Autodesk Inventor part; units mm, degrees
ref_plane "YZ Plane" through (0, 0, 0) normal (1, 0, 0) x (0, 1, 0)
ref_plane "XZ Plane" through (0, 0, 0) normal (0, 1, 0) x (-1, 0, 0)
ref_plane "XY Plane" through (0, 0, 0) normal (0, 0, 1) x (1, 0, 0)
sketch "Sketch1" plane through (0, 0, 0) normal (0, 0, 1) x (1, 0, 0)
  line L0 (0, 39.36) -> (0, -6.56)
  line L1 (-29.4, 0) -> (29.4, 0)
  line L2 (-21, 0) -> (21, 0)
  line L3 (21, 0) -> (21, 6)
  line L4 (21, 6) -> (9, 6)
  line L5 (9, 6) -> (9, 32.8)
  line L6 (9, 32.8) -> (0.5, 32.8)
  line L7 (0.5, 32.8) -> (0.5, 23.9686)
  line L8 (-0.5, 23.9686) -> (-0.5, 32.8)
  line L9 (-0.5, 32.8) -> (-9, 32.8)
  line L10 (-9, 32.8) -> (-9, 6)
  line L11 (-9, 6) -> (-21, 6)
  line L12 (-21, 6) -> (-21, 0)
  circle A0 centre (0, 20) radius 4
  point P0 (0, 0)
  dimension "d0" = 42
  dimension "d1" = 6
  dimension "d2" = 20
  dimension "d3" = 32.8
  dimension "d4" = 21
  dimension "d5" = 18
  dimension "d6" = 8
  dimension "d7" = 1
extrude "Extrusion1" add sketch "Sketch1" along normal mid plane 14 contours A0 L7 L6 L5 L4 L3 L1 L0 | L0 L1 L12 L11 L10 L9 L8 A0
sketch "Sketch2" plane through (-21, 6, -7) normal (0, 1, 0) x (1, 0, 0)
  line L0 (0, 0) -> (12, 0)
  line L1 (0, 0) -> (0, -14)
  line L2 (12, -14) -> (0, -14)
  line L3 (12, 0) -> (12, -14)
  line L4 (30, 0) -> (42, 0)
  line L5 (30, 0) -> (30, -14)
  line L6 (42, -14) -> (30, -14)
  line L7 (42, 0) -> (42, -14)
  circle A0 centre (5, -7) radius 2.75
  circle A1 centre (37, -7) radius 2.75
  line L8 (21, 2.8) -> (21, -16.8)
  line L9 (50.4, -7) -> (-8.4, -7)
  point P0 (21, -7)
  dimension "d10" = 5.5
  dimension "d11" = 32
  dimension "d21" = 5
extrude "Extrusion2" cut sketch "Sketch2" against normal up to next contours L9 A0 | A0 L9 | L9 A1 | A1 L9
sketch "Sketch3" plane through (9, 6, 7) normal (1, 0, 0) x (0, 0, -1)
  line L0 (14, 26.8) -> (0, 26.8)
  line L1 (0, 0) -> (0, 26.8)
  line L2 (14, 0) -> (0, 0)
  line L3 (14, 26.8) -> (14, 0)
  circle A0 centre (7, 22.8) radius 2.75
  line L4 (14, 26.8) -> (0, 26.8) construction
  line L5 (7, 26.8) -> (7, 0) construction
  line L6 (14, 0) -> (0, 0) construction
  point P0 (7, -6)
  dimension "d14" = 5.5
  dimension "d15" = 4
extrude "Extrusion3" cut sketch "Sketch3" against normal up to surface (18 mm away) contours A0
chamfer "Chamfer1" distance 0.5 angle 45 6 edges at (0, 16, 7) (0, 16, -7) (9, 28.8, 2.75) (13.25, 6, 0) (-9, 28.8, 2.75) (-18.75, 6, 0)
properties part number "Linear Rail Shaft Guide" material "Aluminum 6061"
The model under review builds one solid part; all positions refer to its coordinate system, in mm. A direction names the side the tool comes from. Coordinates: 2 decimals unless noted, no trailing zeros. Write each loop counter-clockwise with the first axis right and the second up, starting at its lowest first coordinate (ties: lowest second). Pieces come first, ordered by that corner, then holes.
1) Machinability: for faces 1 (the face through (0.5, 26, -2)), 2 (the face through (12, 6, 0)), 3 (the face through (-12, 6, 0)), which of the approach directions +Z, -Z, +X, -X, +Y, -Y give a long, thin tool a straight path to every point of the face, cutting with its end or side? Answer none if there is none.
2) We need section C-C on x = 16. State the section outline as (y, z) points, then the cut area to 4 significant figures.
3) We need section B-B on y = 20. State the section outline as (x, z) points, then the cut area to 4 significant figures.
4) To check wall thickness, follow probe 1 along X at (y, z) = (1.75, 0); probe 2 along X at (y, z) = (25.5, 6.5); probe 3 along X at (y, z) = (20, -2). State the ranges of each line that lie inside material, in increasing order.
5) We need section A-A on y = 28.8. State the section outline as (x, z) points.
6) The part is to be moulded in two halves that separate along Z. For faces 4 (the face through (0, 9, -7)), 5 (the face through (0, 16, 0)), 6 (the face through (-4.44, 31.12, -1.48)), 7 (the face through (-18.747, 2.788, -0.121)), say which applies: pulls with the +Z half, pulls with the -Z half, needs draft (parallel to the pull), parting line crosses it, or undercut.
7) Clearance check with flat-ended pins moving along their axes: pin 1 Ø1 at (y, z) = (24.5, -0.5) entering from +X; pin 2 Ø6 at (x, z) = (14, 2) entering from +Y; pin 3 Ø3.5 at (x, z) = (16, 0) entering from +Y; pin 4 Ø4 at (y, z) = (14, 1) entering from -X. State where each tip first meets the part, or that it passes through.
8) We need section D-D on z = -4. State the section outline as (x, y) points, then the cut area to 3 significant figures.
Answer list:
1. face 1: +Z, -Z, +Y
1. face 2: +Z, -Z, +X, +Y
1. face 3: +Z, -Z, -X, +Y
2. outline: (0, -7) - (6, -7) - (6, -3.25) - (5.5, -2.75) - (0, -2.75) - close; (0, 2.75) - (5.5, 2.75) - (6, 3.25) - (6, 7) - (0, 7) - close
2. area: 50.75 mm2
3. outline: (-9, -7) - (-4.5, -7) - (-4, -6.5) - (-4, 6.5) - (-4.5, 7) - (-9, 7) - close; (4, -6.5) - (4.5, -7) - (9, -7) - (9, 7) - (4.5, 7) - (4, 6.5) - close
3. area: 139.5 mm2
4. probe 1: x = -21 to -18.75, -13.25 to 13.25, 18.75 to 21
4. probe 2: x = -9 to -0.5, 0.5 to 9
4. probe 3: x = -9 to -4, 4 to 9
5. outline: (-9, -7) - (-0.5, -7) - (-0.5, -2.75) - (-8.5, -2.75) - (-9, -3.25) - close; (-9, 3.25) - (-8.5, 2.75) - (-0.5, 2.75) - (-0.5, 7) - (-9, 7) - close; (0.5, -7) - (9, -7) - (9, -3.25) - (8.5, -2.75) - (0.5, -2.75) - close; (0.5, 2.75) - (8.5, 2.75) - (9, 3.25) - (9, 7) - (0.5, 7) - close
6. face 4: pulls with the -Z half
6. face 5: needs draft
6. face 6: undercut
6. face 7: undercut
7. pin 1: stops at x = 9
7. pin 2: stops at y = 6
7. pin 3: passes through
7. pin 4: stops at x = -9
8. outline: (-21, 0) - (21, 0) - (21, 6) - (9, 6) - (9, 32.8) - (0.5, 32.8) - (0.5, 23.97) arc R4 cw (long way) to (-0.5, 23.97) - (-0.5, 32.8) - (-9, 32.8) - (-9, 6) - (-21, 6) - close
8. area: 675 mm2
